```python
from build123d import *

# Parameters (mm, degrees)
F0_W = 1.5
F0_H = 10


# Not quite as in the source:
# - a fillet or chamfer that OpenCascade refuses, or shapes differently, is made with other operations: its cross-section is extruded or revolved along the edge and cut away or added


with BuildPart() as f1:
    # F0 (on Front) → F1 (revolve)
    with BuildSketch(Plane.XZ):
        Polygon((0, 11.5), (0, 10), (11, 10), (12.5, 10), (17.5, 10), (17.5, 11.5), align=None)
        with Locations((11.75, 5)):
            Rectangle(F0_W, F0_H)
    revolve(axis=Axis((0, 0, 10.75), (0, 0, -1)))

    # F2: chamfer of 2 on 1 edges, made by hand

    # F2_s1 → F2_t2 (revolve, cut)
    with BuildSketch(Plane.XZ):
        Polygon((17.5, 9.5), (15.5, 11.5), (17.5, 11.5), align=None)
    revolve(axis=Axis((0, 0, 11.5), (0, 0, -1)), mode=Mode.SUBTRACT)


solid = f1.part
```
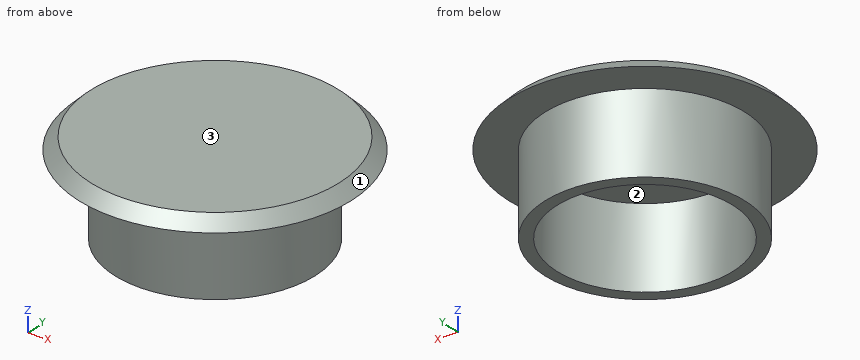
Read the model definition and answer for the solid it produces. Units are mm, in the model's axes. Face numbers are marked on the shaded views. Give positions to 0.01 mm unless a question says otherwise; leave off trailing zeros. Order: outer loops, then holes, each group sorted by start corner. A loop starts at its lowest first (then second) coordinate and runs counter-clockwise, first axis right, second up.
(1) Find section C-C (z = 7.25). Give the vertices of the cut face in (x, y).
(2) Straight lines are drawn through the part: L1, parallel to X at y = 0, z = 3.5; L2, parallel to Z at x = 9, y = 3. For each, find the intervals that lie inside material, in ascending order.
(3) For a pull along X with two mould halves and no side action, classify the marked faces 1, 2 and 3 as released by +X, released by -X, zero draft, split by the parting line, or undercut.
(4) Given pin 1 (5 mm diameter, centred on y = -3.5, z = 7, fed in from +X); pin 2 (1 mm diameter, centred on x = 6, y = 4.5, fed in from -Z); pin 3 (5 mm diameter, centred on y = -10.5, z = 6, fed in from +X), each flat-ended and moving along its own axis, determine where each tip first touches the part or whether it passes through.
(5) Find section A-A (x = 0). Give the vertices of the cut face in (y, z), plus the area to 4 significant figures.
Result sheet:
1. outline: circle Ø25 at (0, 0); hole circle Ø22 at (0, 0)
2. L1: x = -12.5 to -11, 11 to 12.5
2. L2: z = 10 to 11.5
3. face 1: split by the parting line
3. face 2: undercut
3. face 3: zero draft
4. pin 1: stops at x = 12.46
4. pin 2: stops at z = 10
4. pin 3: stops at x = 9.6
5. outline: (-17, 10) - (-12.5, 10) - (-12.5, 0) - (-11, 0) - (-11, 10) - (11, 10) - (11, 0) - (12.5, 0) - (12.5, 10) - (17, 10) - (15.5, 11.5) - (-15.5, 11.5) - close
5. area: 78.75 mm2
